Input: part model. Units: mm. Frame: model coordinates. Face numbers are marked on the shaded views. A direction names the side the tool comes from. Coordinates: 2 decimals unless noted, no trailing zeros. Write each loop counter-clockwise with the first axis right and the second up, starting at its lowest first coordinate (ties: lowest second). Pieces come first, ordered by that corner, then holes. Notation, with made-up numbers: M 2.5,54.25 L 35.5,54.25 A25 ccw 35.5,68.25 Z; hole C 8,-23.75 d6. An arc over 180 degrees is marked long. Write each question's results on one line, items separated by ' | '. Start each with the question number.
1. Set-up query: the marked faces 5, 6, 7, 8 and 9. Return all of +Z, -Z, +X, -X, +Y, -Y with unobstructed straight access to the full face (end or side cutting, diameter ignored); none if empty.
2. Pull-direction query (X, two-part tool) for the marked faces 1, 2, 3 and 4; classes: +X half, -X half, draft (parallel to the pull), parting line (faces both ways), or undercut.
3. First-contact query: pin 1 (0.8 mm diameter, centred on x = 7.5, y = 0.5, fed in from +Z); pin 2 (0.8 mm diameter, centred on x = -7.5, z = 3.5, fed in from -Y); pin 3 (0.5 mm diameter, centred on x = 7.5, z = 4, fed in from +Y); pin 4 (4 mm diameter, centred on x = -3.5, z = 3, fed in from +Y). Flat tips, straight axial feed; report the tip coordinate or a pass-through.
4. Section query C-C, the plane z = 0.25. Count the separate pieces of the cut face and the enclosed holes in it, and give its area (3 significant figures).
5. Section query A-A, the plane z = 3. Output: boundary loops of the cut face in (x, y).
6. Section query B-B, the plane y = 1.25. Output: boundary loops of the cut face in (x, z), and give its area (3 significant figures).
7. Section query D-D, the plane x = -2. Output: boundary loops of the cut face in (y, z).
8. Ray query, probe 1 along Y at (x, z) = (7.5, 4.25); probe 2 along X at (y, z) = (1.5, 5.5); probe 3 along X at (y, z) = (1.5, 2). Return the intervals inside material, ascending.
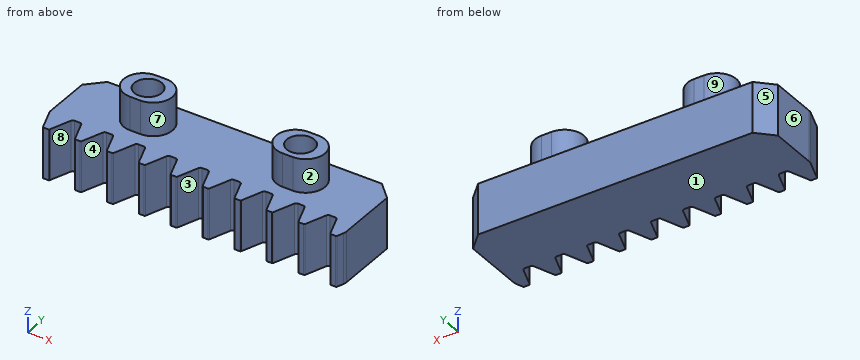
```python
from build123d import *

# Parameters (mm, degrees)
SZKIC1_W                    = 30
SZKIC1_H                    = 8.5
DODANIE_WYCI_GNI_CIE1_DEPTH = 2.5
WYTNIJ_WYCI_GNI_CIE1_DEPTH  = 16.789632675
ZAOKR_GLENIE1_R             = 0.25
ZAOKR_GLENIE2_R             = 0.1
SZYK_START                  = -2.5
SZYK_LINIOWY1_DEPTH         = 5
ZAOKR_GLENIE3_R             = 1
DODANIE_WYCI_GNI_CIE2_DEPTH = 3.3
SZKIC4_R                    = 1.35
WYTNIJ_WYCI_GNI_CIE2_DEPTH  = 7.5
SFAZOWANIE1_SIZE            = 1.5


# Read off the part's stored shape, not the designer's step: Szyk liniowy1
with BuildPart() as part:
    # Szkic1 → Dodanie-wyciągnięcie1 (new, symmetric)
    with BuildSketch(Plane.XY):
        Rectangle(SZKIC1_W, SZKIC1_H)
    extrude(amount=DODANIE_WYCI_GNI_CIE1_DEPTH, both=True)

    # Szkic2 → Wytnij-wyciągnięcie1 (cut, symmetric)
    with BuildSketch(Plane.XY):
        Polygon((-13.57, -4.25), (-12.75, -2), (-11.86, -2), (-11.04, -4.25), align=None)
    extrude(amount=WYTNIJ_WYCI_GNI_CIE1_DEPTH, both=True, mode=Mode.SUBTRACT)

    # Zaokrąglenie1
    zaokr_glenie1_edges = [part.edges().sort_by_distance(p)[0] for p in [
        (-12.75, -2, 0),
        (-11.86, -2, 0),
    ]]
    fillet(zaokr_glenie1_edges, radius=ZAOKR_GLENIE1_R)

    # Zaokrąglenie2
    zaokr_glenie2_edges = [part.edges().sort_by_distance(p)[0] for p in [
        (-11.04, -4.25, 0),
        (-13.57, -4.25, 0),
    ]]
    fillet(zaokr_glenie2_edges, radius=ZAOKR_GLENIE2_R)

    # Szyk liniowy1 outline → Szyk liniowy1 (cut)
    with BuildSketch(Plane.XY.offset(SZYK_START)):
        with BuildLine():
            ThreePointArc((-8.660086567, -2.164396615), (-8.751622667, -2.045181975), (-8.894973903, -2))
            Line((-8.894973903, -2), (-9.435026097, -2))
            ThreePointArc((-9.435026097, -2), (-9.578377333, -2.045181975), (-9.669913433, -2.164396615))
            Line((-9.669913433, -2.164396615), (-10.406034627, -4.184241354))
            ThreePointArc((-10.406034627, -4.184241354), (-10.442649067, -4.23192721), (-10.499989561, -4.25))
            Line((-10.499989561, -4.25), (-7.830010439, -4.25))
            ThreePointArc((-7.830010439, -4.25), (-7.887350933, -4.23192721), (-7.923965373, -4.184241354))
            Line((-7.923965373, -4.184241354), (-8.660086567, -2.164396615))
        make_face()
        with BuildLine():
            ThreePointArc((14.713965373, -4.184241354), (14.677350933, -4.23192721), (14.620010439, -4.25))
            Line((14.620010439, -4.25), (15, -4.25))
            Line((15, -4.25), (15, -3.399390244))
            Line((15, -3.399390244), (14.713965373, -4.184241354))
        make_face()
        with BuildLine():
            ThreePointArc((11.573965373, -4.184241354), (11.537350933, -4.23192721), (11.480010439, -4.25))
            Line((11.480010439, -4.25), (14.149989561, -4.25))
            ThreePointArc((14.149989561, -4.25), (14.092649067, -4.23192721), (14.056034627, -4.184241354))
            Line((14.056034627, -4.184241354), (13.319913433, -2.164396615))
            ThreePointArc((13.319913433, -2.164396615), (13.228377333, -2.045181975), (13.085026097, -2))
            Line((13.085026097, -2), (12.544973903, -2))
            ThreePointArc((12.544973903, -2), (12.401622667, -2.045181975), (12.310086567, -2.164396615))
            Line((12.310086567, -2.164396615), (11.573965373, -4.184241354))
        make_face()
        with BuildLine():
            ThreePointArc((8.433965373, -4.184241354), (8.397350933, -4.23192721), (8.340010439, -4.25))
            Line((8.340010439, -4.25), (11.009989561, -4.25))
            ThreePointArc((11.009989561, -4.25), (10.952649067, -4.23192721), (10.916034627, -4.184241354))
            Line((10.916034627, -4.184241354), (10.179913433, -2.164396615))
            ThreePointArc((10.179913433, -2.164396615), (10.088377333, -2.045181975), (9.945026097, -2))
            Line((9.945026097, -2), (9.404973903, -2))
            ThreePointArc((9.404973903, -2), (9.261622667, -2.045181975), (9.170086567, -2.164396615))
            Line((9.170086567, -2.164396615), (8.433965373, -4.184241354))
        make_face()
        with BuildLine():
            ThreePointArc((5.293965373, -4.184241354), (5.257350933, -4.23192721), (5.200010439, -4.25))
            Line((5.200010439, -4.25), (7.869989561, -4.25))
            ThreePointArc((7.869989561, -4.25), (7.812649067, -4.23192721), (7.776034627, -4.184241354))
            Line((7.776034627, -4.184241354), (7.039913433, -2.164396615))
            ThreePointArc((7.039913433, -2.164396615), (6.948377333, -2.045181975), (6.805026097, -2))
            Line((6.805026097, -2), (6.264973903, -2))
            ThreePointArc((6.264973903, -2), (6.121622667, -2.045181975), (6.030086567, -2.164396615))
            Line((6.030086567, -2.164396615), (5.293965373, -4.184241354))
        make_face()
        with BuildLine():
            ThreePointArc((2.153965373, -4.184241354), (2.117350933, -4.23192721), (2.060010439, -4.25))
            Line((2.060010439, -4.25), (4.729989561, -4.25))
            ThreePointArc((4.729989561, -4.25), (4.672649067, -4.23192721), (4.636034627, -4.184241354))
            Line((4.636034627, -4.184241354), (3.899913433, -2.164396615))
            ThreePointArc((3.899913433, -2.164396615), (3.808377333, -2.045181975), (3.665026097, -2))
            Line((3.665026097, -2), (3.124973903, -2))
            ThreePointArc((3.124973903, -2), (2.981622667, -2.045181975), (2.890086567, -2.164396615))
            Line((2.890086567, -2.164396615), (2.153965373, -4.184241354))
        make_face()
        with BuildLine():
            ThreePointArc((-0.986034627, -4.184241354), (-1.022649067, -4.23192721), (-1.079989561, -4.25))
            Line((-1.079989561, -4.25), (1.589989561, -4.25))
            ThreePointArc((1.589989561, -4.25), (1.532649067, -4.23192721), (1.496034627, -4.184241354))
            Line((1.496034627, -4.184241354), (0.759913433, -2.164396615))
            ThreePointArc((0.759913433, -2.164396615), (0.668377333, -2.045181975), (0.525026097, -2))
            Line((0.525026097, -2), (-0.015026097, -2))
            ThreePointArc((-0.015026097, -2), (-0.158377333, -2.045181975), (-0.249913433, -2.164396615))
            Line((-0.249913433, -2.164396615), (-0.986034627, -4.184241354))
        make_face()
        with BuildLine():
            ThreePointArc((-4.126034627, -4.184241354), (-4.162649067, -4.23192721), (-4.219989561, -4.25))
            Line((-4.219989561, -4.25), (-1.550010439, -4.25))
            ThreePointArc((-1.550010439, -4.25), (-1.607350933, -4.23192721), (-1.643965373, -4.184241354))
            Line((-1.643965373, -4.184241354), (-2.380086567, -2.164396615))
            ThreePointArc((-2.380086567, -2.164396615), (-2.471622667, -2.045181975), (-2.614973903, -2))
            Line((-2.614973903, -2), (-3.155026097, -2))
            ThreePointArc((-3.155026097, -2), (-3.298377333, -2.045181975), (-3.389913433, -2.164396615))
            Line((-3.389913433, -2.164396615), (-4.126034627, -4.184241354))
        make_face()
        with BuildLine():
            ThreePointArc((-7.266034627, -4.184241354), (-7.302649067, -4.23192721), (-7.359989561, -4.25))
            Line((-7.359989561, -4.25), (-4.690010439, -4.25))
            ThreePointArc((-4.690010439, -4.25), (-4.747350933, -4.23192721), (-4.783965373, -4.184241354))
            Line((-4.783965373, -4.184241354), (-5.520086567, -2.164396615))
            ThreePointArc((-5.520086567, -2.164396615), (-5.611622667, -2.045181975), (-5.754973903, -2))
            Line((-5.754973903, -2), (-6.295026097, -2))
            ThreePointArc((-6.295026097, -2), (-6.438377333, -2.045181975), (-6.529913433, -2.164396615))
            Line((-6.529913433, -2.164396615), (-7.266034627, -4.184241354))
        make_face()
        with BuildLine():
            Line((-15, -4.25), (-14.110010439, -4.25))
            ThreePointArc((-14.110010439, -4.25), (-14.167350933, -4.23192721), (-14.203965373, -4.184241354))
            Line((-14.203965373, -4.184241354), (-14.940086567, -2.164396615))
            ThreePointArc((-14.940086567, -2.164396615), (-14.964838585, -2.11456312), (-15, -2.071438713))
            Line((-15, -2.071438713), (-15, -4.25))
        make_face()
    extrude(amount=SZYK_LINIOWY1_DEPTH, mode=Mode.SUBTRACT)

    # Zaokrąglenie3
    zaokr_glenie3_edges = [part.edges().sort_by_distance(p)[0] for p in [
        (-15, -2.071438713, 0),
        (15, -3.399390244, 0),
    ]]
    fillet(zaokr_glenie3_edges, radius=ZAOKR_GLENIE3_R)

    # Szkic3 → Dodanie-wyciągnięcie2 (add)
    with BuildSketch(Plane.XY.offset(2.5)):
        with BuildLine():
            Line((-8, 3.15), (-7, 3.15))
            ThreePointArc((-7, 3.15), (-5.1, 1.25), (-7, -0.65))
            Line((-7, -0.65), (-8, -0.65))
            ThreePointArc((-8, -0.65), (-9.9, 1.25), (-8, 3.15))
        make_face()
    dodanie_wyci_gni_cie2 = extrude(amount=DODANIE_WYCI_GNI_CIE2_DEPTH)

    # Szkic4 → Wytnij-wyciągnięcie2 (cut)
    with BuildSketch(Plane.XY.offset(5.8)):
        with Locations((-7.5, 1.25)):
            Circle(SZKIC4_R)
    wytnij_wyci_gni_cie2 = extrude(amount=-WYTNIJ_WYCI_GNI_CIE2_DEPTH, mode=Mode.SUBTRACT)

    # Lustro1: Dodanie-wyciągnięcie2, Wytnij-wyciągnięcie2 across plane
    add(dodanie_wyci_gni_cie2.mirror(Plane(origin=(0, 0, 0), x_dir=(0, 0, 1), z_dir=(1, 0, 0))))
    add(wytnij_wyci_gni_cie2.mirror(Plane(origin=(0, 0, 0), x_dir=(0, 0, 1), z_dir=(1, 0, 0))), mode=Mode.SUBTRACT)

    # Sfazowanie1
    sfazowanie1_edges = [part.edges().sort_by_distance(p)[0] for p in [
        (-15, 4.25, 0),
        (15, 4.25, 0),
    ]]
    chamfer(sfazowanie1_edges, length=SFAZOWANIE1_SIZE)


solid = part.part
```
Answer:
1) face 5: +Z, -Z, -X, +Y | face 6: +Z, -Z, -X, +Y, -Y | face 7: +Z | face 8: +Z, -Z, -Y | face 9: +Z, -X
2) face 1: draft | face 2: +X half | face 3: undercut | face 4: undercut
3) pin 1: z = -1.7 | pin 2: y = -0.65 | pin 3: y = 3.15 | pin 4: y = 4.25
4) separate pieces: 1 | enclosed holes: 2 | area: 206 mm^2
5) outline: M -8,-0.65 L -7,-0.65 A1.9 ccw -7,3.15 L -8,3.15 A1.9 ccw Z; M 7,-0.65 L 8,-0.65 A1.9 ccw 8,3.15 L 7,3.15 A1.9 ccw Z; hole C -7.5,1.25 d2.7; hole C 7.5,1.25 d2.7
6) outline: M -15,-2.5 L 15,-2.5 L 15,2.5 L 9.9,2.5 L 9.9,5.8 L 8.85,5.8 L 8.85,-1.7 L 6.15,-1.7 L 6.15,5.8 L 5.1,5.8 L 5.1,2.5 L -5.1,2.5 L -5.1,5.8 L -6.15,5.8 L -6.15,-1.7 L -8.85,-1.7 L -8.85,5.8 L -9.9,5.8 L -9.9,2.5 L -15,2.5 Z | area: 141 mm^2
7) outline: M -3.21,-2.5 L 4.25,-2.5 L 4.25,2.5 L -3.21,2.5 Z
8) probe 1: -0.65 to -0.1, 2.6 to 3.15 | probe 2: -9.88 to -8.83, -6.17 to -5.12, 5.12 to 6.17, 8.83 to 9.88 | probe 3: -15 to -8.83, -6.17 to 6.17, 8.83 to 15
